from build123d import *

# Parameters (mm, degrees)
F1_DEPTH = 28.8


with BuildPart() as f1:
    # F0 (on Top) → F1 (new body, symmetric)
    with BuildSketch(Plane.XY):
        with BuildLine():
            Line((24.2, 15), (7, 15))
            ThreePointArc((7, 15), (2.0502525317, 12.9497474683), (0, 8))
            Line((0, 8), (0, 0))
            Line((0, 0), (31.2, 0))
            Line((31.2, 0), (31.2, 8))
            ThreePointArc((31.2, 8), (29.1497474683, 12.9497474683), (24.2, 15))
        make_face()
    extrude(amount=F1_DEPTH, both=True)


solid = f1.part
Source: CAD feature listing. Evaluate the final solid. Frame: model axes, mm. Give positions to 0.01 mm unless a question says otherwise; leave off trailing zeros. Order: outer loops, then holes, each group sorted by start corner. A loop starts at its lowest first (then second) coordinate and runs counter-clockwise, first axis right, second up. Notation, with made-up numbers: (-4.75, 48) -> (11.25, 48) arc R20 ccw to (11.25, 74) -> close; hole circle Ø2 at (-34.75, 71.5). An arc over 180 degrees is marked (long way). Use a Markdown table: item, result.
1) Section query A-A, the plane z = 2. Return the cut outline in (x, y).
Answer list:
| item | result |
|---|---|
| outline | (0, 0) -> (31.2, 0) -> (31.2, 8) arc R7 ccw to (24.2, 15) -> (7, 15) arc R7 ccw to (0, 8) -> close |
2) Mould query, pull axis Z, two halves, no side actions, for faces 1 (the flat face through (16, 15, 0)), 2 (the flat face through (15, 8, -28.8)), 3 (the flat face through (15, 8, 28.8)). Classes: +Z half, -Z half, draft (parallel to the pull), parting line (faces both ways), or undercut.
Answer list:
| item | result |
|---|---|
| face 1 | draft |
| face 2 | -Z half |
| face 3 | +Z half |
3) Section query B-B, the plane x = 26. Return the cut outline in (y, z), then the cut area to 3 significant figures.
Answer list:
| item | result |
|---|---|
| outline | (0, -28.8) -> (14.76, -28.8) -> (14.76, 28.8) -> (0, 28.8) -> close |
| area | 850 mm² |
4) Ray query, line 1 along Y through (x, z) = (27, -10.5); line 2 along X through (y, z) = (14.25, -1.5); line 3 along X through (y, z) = (9.25, 13.5). Return the intervals inside material, ascending. Write a range as [from, to].
Answer list:
| item | result |
|---|---|
| line 1 | [0, 14.42] |
| line 2 | [3.85, 27.35] |
| line 3 | [0.11, 31.09] |
